The listing builds one solid part. Answer for the finished solid, in the listing's coordinates (mm). Face numbers are marked on the shaded views. A direction names the side the tool comes from. Coordinates: 2 decimals unless noted, no trailing zeros. Write each loop counter-clockwise with the first axis right and the second up, starting at its lowest first coordinate (ties: lowest second). Pieces come first, ordered by that corner, then holes.
from build123d import *

# Parameters (mm, degrees)
F2_R     = 0.5
F3_DEPTH = 25
F4_R     = 0.3


with BuildPart() as f1:
    # F0 (on Front) → F1 (revolve)
    with BuildSketch(Plane.XZ):
        Polygon((0, 1), (0, 0), (5, 0), (5, 4), (1, 4), (1, 1), align=None)
    revolve(axis=Axis((2.5, 0, 0), (-1, 0, 0)))

    # F2 (on Right) → F3 (intersect)
    with BuildSketch(Plane.YZ):
        with BuildLine():
            Line((4.000914, 0.006655), (1, 0))
            Line((1, 0), (0.995769, 1.908105))
            ThreePointArc((0.995769, 1.908105), (0, 3), (-0.995769, 1.908105))
            Line((-0.995769, 1.908105), (-1, 0))
            Line((-1, 0), (-4.000914, 0.006655))
            ThreePointArc((-4.000914, 0.006655), (0, -4.000919), (4.000914, 0.006655))
        make_face()
        Circle(F2_R, mode=Mode.SUBTRACT)
        with Locations((0, 2)):
            Circle(F2_R, mode=Mode.SUBTRACT)
    extrude(amount=F3_DEPTH, mode=Mode.INTERSECT)

    # F4
    f4_edges = [f1.edges().sort_by_distance(p)[0] for p in [
        (3, -3.999994, 0.006653),
        (3, 3.999994, 0.006653),
        (0, 0.999995, 0.002218),
    ]]
    fillet(f4_edges, radius=F4_R)


solid = f1.part
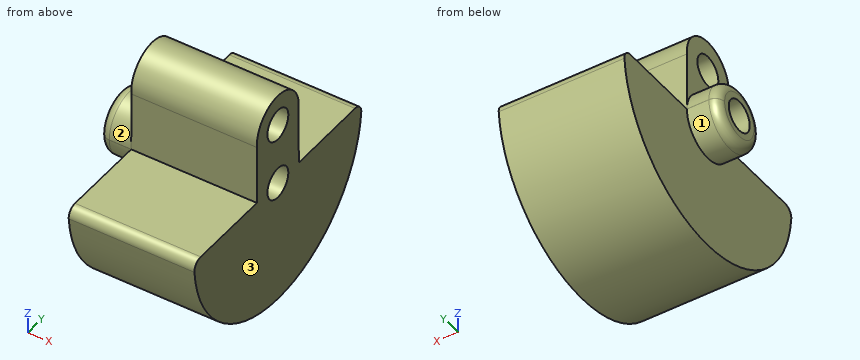
Q1. Given pin 1 (1 mm diameter, centred on x = 4, y = -3, fed in from -Z); pin 2 (2 mm diameter, centred on y = 0.5, z = -3, fed in from -X), each flat-ended and moving along its own axis, determine where each tip first touches the part or whether it passes through.
Answers below:
pin 1: stops at z = -3.12
pin 2: stops at x = 1
Q2. Find the intervals of material crossed by probe 1 along Z at (x, y) = (3.15, 0); probe 2 along Y at (x, z) = (3, 2); probe 3 along X at (y, z) = (1.75, -3.5), in increasing order.
Answers below:
probe 1: z = -4 to -0.5, 0.5 to 1.5, 2.5 to 3
probe 2: y = -1 to -0.5, 0.5 to 1
probe 3: x = 1 to 5
Q3. The part is cut by section B-B, the plane x = 2.05. Write down the section's boundary in (y, z).
Answers below:
outline: (-3.99, -0.32) arc R4 ccw to (3.99, -0.32) arc R0.3 ccw to (3.69, 0.01) - (1, 0) - (1, 1.91) arc R1 ccw (long way) to (-1, 1.91) - (-1, 0) - (-3.69, 0.01) arc R0.3 ccw to start; hole circle Ø1 at (0, 0); hole circle Ø1 at (0, 2)
Q4. Which of the six approach directions +Z, -Z, +X, -X, +Y, -Y give full straight-line access (tool end or side, diameter ignored) to the marked faces 1, 2 and 3?
Answers below:
face 1: -Z, -X
face 2: +Z, -X
face 3: +Z, -Z, +X, +Y, -Y
Q5. The part is cut by section C-C, the plane z = 2.25. Write down the section's boundary in (x, y).
Answers below:
outline: (1, -0.97) - (5, -0.97) - (5, -0.43) - (1, -0.43) - close; (1, 0.43) - (5, 0.43) - (5, 0.97) - (1, 0.97) - close
Q6. The part is cut by section D-D, the plane z = -2.25. Write down the section's boundary in (x, y).
Answers below:
outline: (1, -3.31) - (5, -3.31) - (5, 3.31) - (1, 3.31) - close
Q7. The part is cut by section A-A, the plane y = 0. Write down the section's boundary in (x, z).
Answers below:
outline: (0, -0.7) arc R0.3 ccw to (0.3, -1) - (1, -1) - (1, -4) - (5, -4) - (5, -0.5) - (0, -0.5) - close; (0, 0.5) - (5, 0.5) - (5, 1.5) - (1, 1.5) - (1, 1) - (0.3, 1) arc R0.3 ccw to (0, 0.7) - close; (1, 2.5) - (5, 2.5) - (5, 3) - (1, 3) - close
